Job drawing, mm, ordinate dimensions from the low corner. One solid piece. A direction names the side the tool comes from. Round coordinates to 2 decimals unless told otherwise and drop trailing zeros. Loops run counter-clockwise (first coordinate to the right, second up) from the corner with the lowest first, then second, coordinate; pieces in that order, holes last.
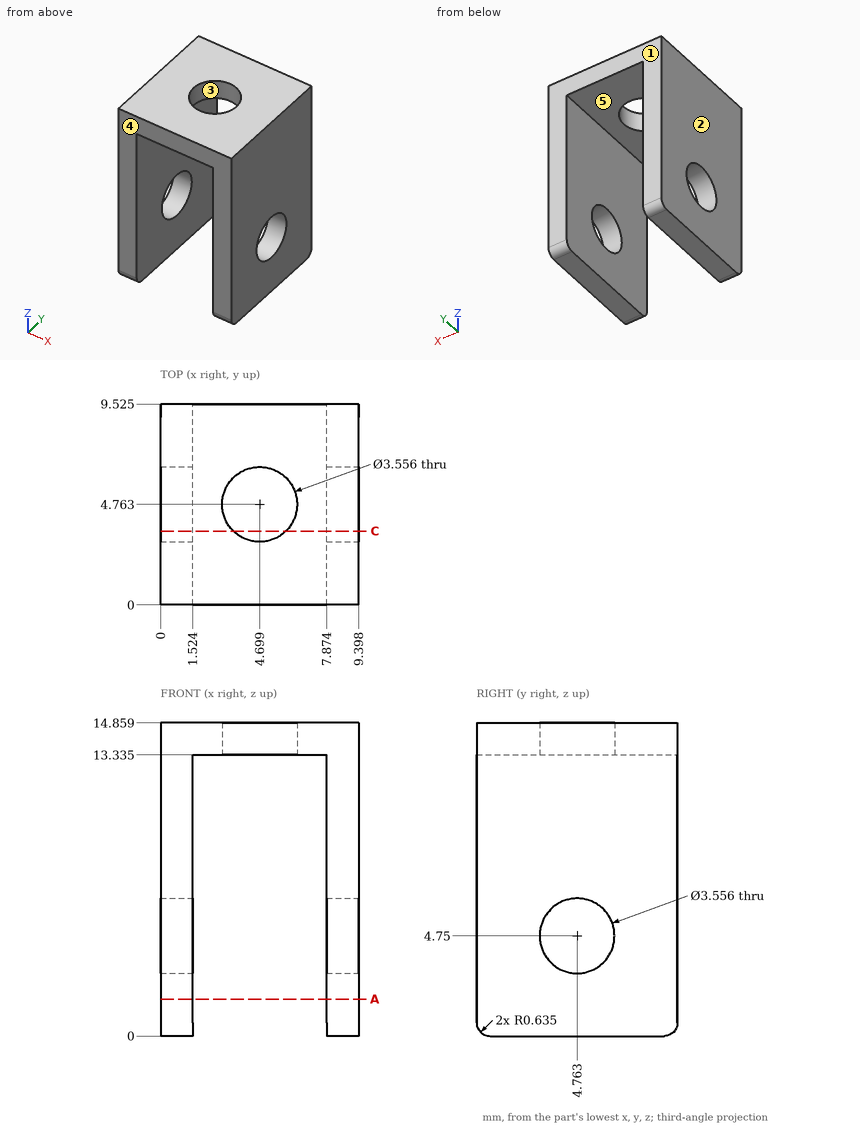
(1) Which spindle directions (+Z, -Z, +X, -X, +Y, -Y) get a long thin tool onto all of the face, cutting with end or side? Do the marked faces 4 and 5. Say none if no direction does.
Responses:
face 4: +Z, -Z, +X, -X, -Y
face 5: -Z, +Y, -Y
(2) Slice it at C-C on y = 3.5. Count the separate pieces of the cut face and the enclosed holes in it.
Responses:
separate pieces: 4
enclosed holes: 0
(3) Slice it at A-A on z = 1.75. List the corners of the cut face in (x, y) (1 decimal).
Responses:
outline: (0, 0) - (1.5, 0) - (1.5, 9.5) - (0, 9.5) - close; (7.9, 0) - (9.4, 0) - (9.4, 9.5) - (7.9, 9.5) - close
(4) Pin check, flat tips, straight feed: P1, Ø1.9, axis at x = 3, y = 4, coming from the -Z side (1 decimal); P2, Ø4, axis at x = 5.5, z = 2.5, coming from the -Y side. Stop position of each tip, or through.
Responses:
P1: stops at z = 13.3
P2: passes through
(5) Probe line 1 (X direction, y = 7.25, z = 7.5) (1 decimal); line 2 (Z direction, x = 6.25, y = 3) (1 decimal); line 3 (Y direction, x = 0.75, z = 5.75) (1 decimal). List the from-to ranges inside material, lowest first.
Responses:
line 1: x = 0 to 1.5, 7.9 to 9.4
line 2: z = 13.3 to 14.9
line 3: y = 0 to 3.3, 6.2 to 9.5
(6) Pull direction X, two halves, no side cores. Call the marked faces 1, 2 and 3: +X half, -X half, draft (parallel to the pull), parting line (faces both ways), or undercut.
Responses:
face 1: draft
face 2: -X half
face 3: undercut
